Source: CAD feature listing. Evaluate the final solid. Frame: model axes, mm. A direction names the side the tool comes from. Round coordinates to 2 decimals unless told otherwise and drop trailing zeros. Write each loop counter-clockwise with the first axis right and the second up, starting at its lowest first coordinate (ties: lowest second). Pieces come first, ordered by that corner, then holes. Notation, with made-up numbers: (68, -28) -> (87, -28) arc R25 ccw to (87, 7) -> close; hole circle Ø6 at (28, 10.5). An arc over 180 degrees is marked (long way). Put each result on its own line as item: value.
```python
from build123d import *

# Parameters (mm, degrees)
BOSS_EXTRU_1_DEPTH      = 2
CONG_2_R                = 1.35
ESQUISSE4_R             = 0.75
ENL_V_MAT_EXTRU_2_DEPTH = 176.894862906
CONG_5_R                = 1
ENL_V_MAT_EXTRU_3_DEPTH = 4
CONG_3_R                = 2.5
CONG_4_R                = 0.8


with BuildPart() as part:
    # Esquisse2 → Boss.-Extru.1 (new body)
    with BuildSketch(Plane(origin=(0, 0, 0), x_dir=(0, 0, -1), z_dir=(1, 0, 0))):
        with BuildLine():
            Line((0, 0), (170.873171093, 0))
            ThreePointArc((170.873171093, 0), (174.177922559, 2.347343181), (173.049882129, 6.240789861))
            ThreePointArc((173.049882129, 6.240789861), (150.444362328, 18.689979585), (125, 23))
            ThreePointArc((125, 23), (61.450806457, 17.202138822), (0, 0))
        make_face()
    extrude(amount=BOSS_EXTRU_1_DEPTH)

    # Congé2
    cong_2_edges = [part.edges().sort_by_distance(p)[0] for p in [
        (1, 0, 0),
    ]]
    fillet(cong_2_edges, radius=CONG_2_R)

    # Esquisse4 → Enlèv. mat.-Extru.2 (cut, through all)
    with BuildSketch(Plane(origin=(2, 0, 0), x_dir=(0, 0, -1), z_dir=(1, 0, 0))):
        with BuildLine():
            ThreePointArc((125.75, 21.2), (125.632543584, 21.602974706), (125.316963696, 21.87973084))
            Line((125.316963696, 21.87973084), (125, 21.2))
            Line((125, 21.2), (124.683036304, 21.87973084))
            ThreePointArc((124.683036304, 21.87973084), (124.597025294, 20.567456416), (125.75, 21.2))
        make_face()
        with BuildLine():
            Line((125, 21.2), (125.316963696, 21.87973084))
            ThreePointArc((125.316963696, 21.87973084), (125, 21.95), (124.683036304, 21.87973084))
            Line((124.683036304, 21.87973084), (125, 21.2))
        make_face()
        with Locations((172.368958832, 3.328337296)):
            Circle(ESQUISSE4_R)
        with Locations((9.5, 1.731368161)):
            Circle(ESQUISSE4_R)
        with BuildLine():
            Line((125.316963696, 21.87973084), (125.837238378, 22.995463495))
            ThreePointArc((125.837238378, 22.995463495), (125.418625334, 22.998865865), (125, 23))
            ThreePointArc((125, 23), (124.580556422, 22.999749507), (124.161113442, 22.99899803))
            Line((124.161113442, 22.99899803), (124.683036304, 21.87973084))
            ThreePointArc((124.683036304, 21.87973084), (125, 21.95), (125.316963696, 21.87973084))
        make_face()
        with BuildLine():
            Line((125.837238378, 22.995463495), (126.398922974, 24.2))
            Line((126.398922974, 24.2), (123.601077026, 24.2))
            Line((123.601077026, 24.2), (124.161113442, 22.99899803))
            ThreePointArc((124.161113442, 22.99899803), (124.580556422, 22.999749507), (125, 23))
            ThreePointArc((125, 23), (125.418625334, 22.998865865), (125.837238378, 22.995463495))
        make_face()
        with BuildLine():
            ThreePointArc((174.217111681, 2.466529469), (174.369594573, 3.34181388), (174.296772549, 4.227291596))
            Line((174.296772549, 4.227291596), (173.048689672, 3.645300993))
            ThreePointArc((173.048689672, 3.645300993), (173.101180837, 3.490667007), (173.118958832, 3.328337296))
            ThreePointArc((173.118958832, 3.328337296), (173.101180837, 3.166007586), (173.048689672, 3.0113736))
            Line((173.048689672, 3.0113736), (174.217111681, 2.466529469))
        make_face()
        with BuildLine():
            ThreePointArc((173.118958832, 3.328337296), (173.101180837, 3.490667007), (173.048689672, 3.645300993))
            Line((173.048689672, 3.645300993), (172.368958832, 3.328337296))
            Line((172.368958832, 3.328337296), (173.048689672, 3.0113736))
            ThreePointArc((173.048689672, 3.0113736), (173.101180837, 3.166007586), (173.118958832, 3.328337296))
        make_face()
        with BuildLine():
            Line((172.368958832, 3.328337296), (173.048689672, 3.645300993))
            ThreePointArc((173.048689672, 3.645300993), (171.618958832, 3.328337296), (173.048689672, 3.0113736))
            Line((173.048689672, 3.0113736), (172.368958832, 3.328337296))
        make_face()
        with BuildLine():
            Line((175.368958832, 4.727260271), (174.296772549, 4.227291596))
            ThreePointArc((174.296772549, 4.227291596), (174.369594573, 3.34181388), (174.217111681, 2.466529469))
            Line((174.217111681, 2.466529469), (175.368958832, 1.929414322))
            Line((175.368958832, 1.929414322), (175.368958832, 4.727260271))
        make_face()
        with BuildLine():
            ThreePointArc((9.183036304, 1.051637321), (9.5, 0.981368161), (9.816963696, 1.051637321))
            Line((9.816963696, 1.051637321), (9.5, 1.731368161))
            Line((9.5, 1.731368161), (9.183036304, 1.051637321))
        make_face()
        with BuildLine():
            Line((9.5, 1.731368161), (9.816963696, 1.051637321))
            ThreePointArc((9.816963696, 1.051637321), (10.132543584, 1.328393455), (10.25, 1.731368161))
            ThreePointArc((10.25, 1.731368161), (9.097025294, 2.363911745), (9.183036304, 1.051637321))
            Line((9.183036304, 1.051637321), (9.5, 1.731368161))
        make_face()
        with BuildLine():
            Line((8.692649767, 0), (10.307350233, 0))
            Line((10.307350233, 0), (9.816963696, 1.051637321))
            ThreePointArc((9.816963696, 1.051637321), (9.5, 0.981368161), (9.183036304, 1.051637321))
            Line((9.183036304, 1.051637321), (8.692649767, 0))
        make_face()
        Polygon((10.898922974, -1.268631839), (10.307350233, 0), (8.692649767, 0), (8.101077026, -1.268631839), align=None)
    extrude(amount=-ENL_V_MAT_EXTRU_2_DEPTH, mode=Mode.SUBTRACT)

    # Congé5
    cong_5_edges = [part.edges().sort_by_distance(p)[0] for p in [
        (1, 22.99899803, -124.161113442),
        (1, 22.995463495, -125.837238378),
        (1, 4.227291596, -174.296772549),
        (1, 2.466529469, -174.217111681),
        (1, 0, -10.307350233),
        (1, 0, -8.692649767),
    ]]
    fillet(cong_5_edges, radius=CONG_5_R)

    # Esquisse9 → Enlèv. mat.-Extru.3 (cut)
    with BuildSketch(Plane(origin=(0, 0, 0), x_dir=(0, 0, -1), z_dir=(1, 0, 0))):
        with BuildLine():
            Line((126.213985158, 1.761191042), (171.208548293, 1.761191042))
            ThreePointArc((171.208548293, 1.761191042), (170.45940521, 3.723438508), (171.92571116, 5.227292667))
            ThreePointArc((171.92571116, 5.227292667), (150.407492919, 17.120662481), (126.213985158, 21.497892659))
            Line((126.213985158, 21.497892659), (126.213985158, 1.761191042))
        make_face()
        with BuildLine():
            Line((11.749802346, 1.761191042), (60, 1.761191042))
            Line((60, 1.761191042), (60, 15.113262564))
            ThreePointArc((60, 15.113262564), (35.626415593, 9.474190858), (11.71850292, 2.106527851))
            ThreePointArc((11.71850292, 2.106527851), (11.740815112, 1.934463297), (11.749802346, 1.761191042))
        make_face()
        with BuildLine():
            Line((61.5, 1.761191042), (123.786014842, 1.761191042))
            Line((123.786014842, 1.761191042), (123.786014842, 21.497892659))
            ThreePointArc((123.786014842, 21.497892659), (92.506301163, 19.845888558), (61.5, 15.400790857))
            Line((61.5, 15.400790857), (61.5, 1.761191042))
        make_face()
    extrude(amount=ENL_V_MAT_EXTRU_3_DEPTH, mode=Mode.SUBTRACT)

    # Congé3
    cong_3_edges = [part.edges().sort_by_distance(p)[0] for p in [
        (1, 15.113262564, -60),
        (1, 21.497892659, -126.213985158),
        (1, 21.497892659, -123.786014842),
        (1, 15.400790857, -61.5),
    ]]
    fillet(cong_3_edges, radius=CONG_3_R)

    # Congé4
    cong_4_edges = [part.edges().sort_by_distance(p)[0] for p in [
        (1, 5.227292667, -171.92571116),
        (1, 1.761191042, -171.208548293),
    ]]
    fillet(cong_4_edges, radius=CONG_4_R)


solid = part.part
```
Q1. Cut plane B-B on z = -25. Output: boundary loops of the cut face in (x, y).
Ans:
outline: (0, 0) -> (2, 0) -> (2, 1.76) -> (0, 1.76) -> close; (0, 6.43) -> (2, 6.43) -> (2, 8.46) -> (0, 8.46) -> close
Q2. Draft query along Z for faces 3 (the cylindrical face through (0.99, 9.16, -34.47)), 4 (the cylindrical face through (0.99, 18.32, -151.48)), 5 (the cylindrical face through (0.986, 19.863, -92.685)), 6 (the cylindrical face through (0.986, 17.884, -65.272)). Return one class per face: +Z half, -Z half, draft (parallel to the pull), parting line (faces both ways), or undercut.
Ans:
face 3: undercut
face 4: -Z half
face 5: undercut
face 6: +Z half
Q3. Cut plane C-C on x = 0.45. Give the number of separate pieces and of enclosed holes in the cut face, and give its area (3 significant figures).
Ans:
separate pieces: 1
enclosed holes: 3
area: 658 mm^2
Q4. Reachability of faces 1 (the flat face through (2, 0.5, -89.7)), 2 (the cylindrical face through (0.99, 16.77, -151.37)) from +Z, -Z, +X, -X, +Y, -Y: full face, straight path, thin tool, end or side. Return the list, or none.
Ans:
face 1: +Z, -Z, +X, +Y, -Y
face 2: +X, -X
Q5. Pin query (flat end, axial travel): pin 1 (0.6 mm diameter, centred on x = 1, z = -27.5, fed in from +Y); pin 2 (0.6 mm diameter, centred on x = 1.5, y = 10.5, fed in from -Z). Return the tip coordinate at first contact, or that it passes through.
Ans:
pin 1: stops at y = 9.28
pin 2: stops at z = -167.59
Q6. Material intervals for line 1 (Z direction, x = 1.65, y = 2); line 2 (Y direction, x = 1.4, z = -125); line 3 (Y direction, x = 0.7, z = -15.5), sorted ascending. Write a range as [from, to].
Ans:
line 1: z = [-173.87, -170.3], [-126.21, -123.79], [-61.5, -60], [-11.73, -10.2], [-8.8, -6.38]
line 2: y = [0, 20.45]
line 3: y = [0, 1.76], [3.4, 5.49]
Q7. Cut plane A-A on z = -95.5. Output: boundary loops of the cut face in (x, y).
Ans:
outline: (0, 0) -> (2, 0) -> (2, 1.76) -> (0, 1.76) -> close; (0, 20.13) -> (2, 20.13) -> (2, 21.76) -> (0, 21.76) -> close
